Here's the drawing with two shaded views (mm, measured from the low corner). I have some questions. A direction names the side the tool comes from. Give positions to 0.01 mm unless a question says otherwise; leave off trailing zeros. Loops run counter-clockwise (first coordinate to the right, second up) from the corner with the lowest first, then second, coordinate; pieces in that order, holes last. Notation, with made-up numbers: (1, -40) - (45, -40) arc R19 cw to (45, -34) - close; hole circle Ø6 at (-15.75, 87.25). An arc over 180 degrees is marked (long way). Answer as a JSON object with one key per item and string values. Group by question number.
Item 1: Which directions (+Z, -Z, +X, -X, +Y, -Y) give clear straight access to the entire face, cutting with the end or side of a thin tool? Please do the marked faces 1 and 2.
Item 2: Please list where this line runs through material, in increasing order: L1, parallel to Z at x = 17, y = 35.
Item 3: Suppose I cut it at C-C on y = 7. Write out the boundary of the cut face in (x, z).
Item 4: Will this pin go through, and if not, where does the flat tip stop? pin 1 (10 mm diameter, centred on x = 33.5, y = 30.5, fed in from -Z).
Item 5: Suppose I cut it at A-A on x = 21. Write out the boundary of the cut face in (y, z).
Item 6: Suppose I cut it at B-B on z = 41. Write out the boundary of the cut face in (x, y), and give its area (3 significant figures).
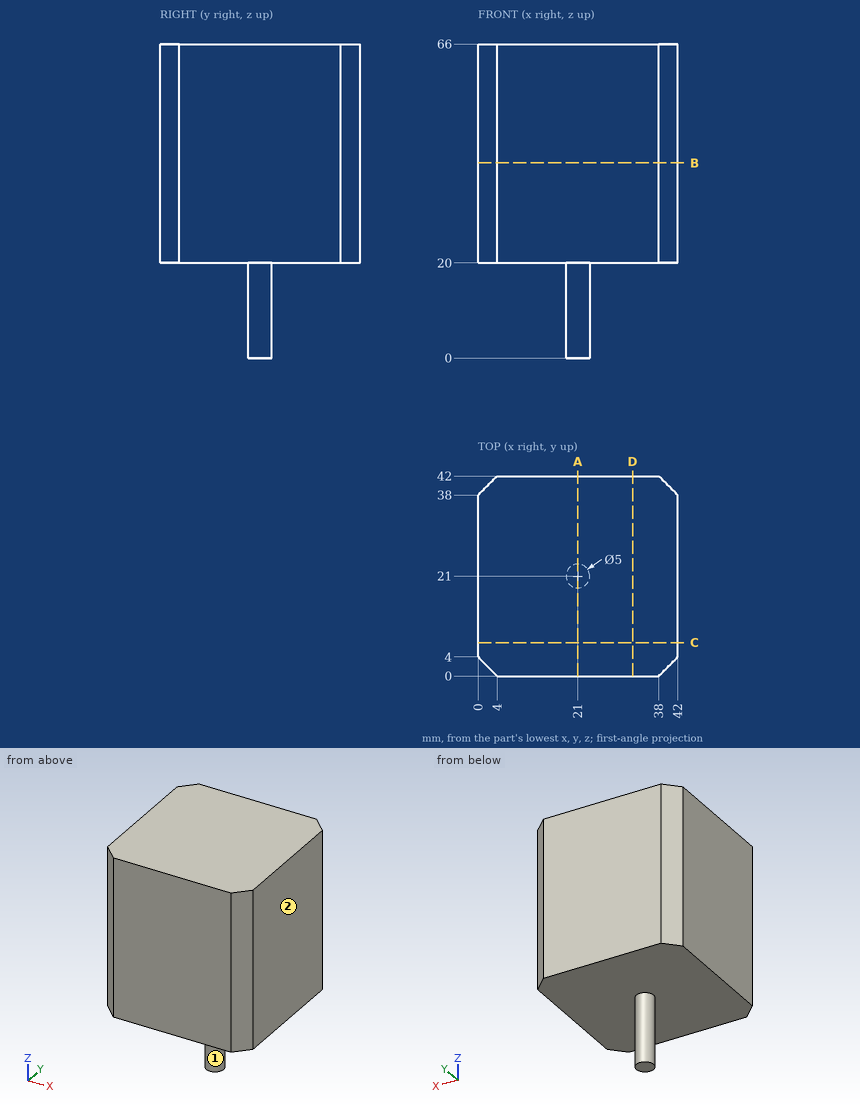
Worked out:
{
 "1": {"face 1": "-Z", "face 2": "+Z, -Z, +X, +Y, -Y"},
 "2": {"L1": "z = 20 to 66"},
 "3": {"outline": "(0, 20) - (42, 20) - (42, 66) - (0, 66) - close"},
 "4": {"pin 1": "stops at z = 20"},
 "5": {"outline": "(0, 20) - (18.5, 20) - (18.5, 0) - (23.5, 0) - (23.5, 20) - (42, 20) - (42, 66) - (0, 66) - close"},
 "6": {"outline": "(0, 4) - (4, 0) - (38, 0) - (42, 4) - (42, 38) - (38, 42) - (4, 42) - (0, 38) - close", "area": "1,730 mm2"}
}
